Part model, mm, in its own coordinate system. A direction names the side the tool comes from. Give positions to 0.01 mm unless a question says otherwise; leave off trailing zeros. Order: outer loops, then holes, each group sorted by start corner. A loop starts at its lowest first (then second) coordinate and runs counter-clockwise, first axis right, second up. Notation, with made-up numbers: (35, -30.75) - (92, -30.75) arc R10 ccw to (92, -17.75) - close; hole circle Ø3 at (-34, 10). An arc over 180 degrees is marked (long way). One line per item, written item: value.
```python
from build123d import *

# Parameters (mm, degrees)
SKETCH1_R           = 140
BOSS_EXTRUDE1_DEPTH = 300
FILLET1_R           = 4


# Read off the part's stored shape, not the designer's step: Shell1
with BuildPart() as part:
    # Sketch1 → Boss-Extrude1 (new body)
    with BuildSketch(Plane(origin=(0, 0, 0), x_dir=(1, 0, 0), z_dir=(0, 1, 0))):
        with Locations(Location((0, 0, 0), (0, 0, 270))):
            Circle(SKETCH1_R)
    extrude(amount=BOSS_EXTRUDE1_DEPTH)

    # Sketch3 → Cut-Revolve1 (revolve, cut)
    with BuildSketch(Plane.XY, mode=Mode.PRIVATE) as cut_revolve1_sk:
        with BuildLine():
            Line((-107.848101266, -4.321058688), (-131.736864002, 293.320012156))
            ThreePointArc((-131.736864002, 293.320012156), (-133.011114968, 295.939391827), (-135.72404248, 297))
            Line((-135.72404248, 297), (-179.746835443, 297))
            Line((-179.746835443, 297), (-193.472957422, -4.321058688))
            Line((-193.472957422, -4.321058688), (-107.848101266, -4.321058688))
        make_face()
    revolve(cut_revolve1_sk.sketch.rotate(Axis((0, -4.321058688, 0), (0, 1, 0)), 270), axis=Axis((0, -4.321058688, 0), (0, 1, 0)), mode=Mode.SUBTRACT)

    # Fillet1
    fillet1_edges = [part.edges().sort_by_distance(p)[0] for p in [
        (0, 0, 108.194910748),
    ]]
    fillet(fillet1_edges, radius=FILLET1_R)

    # Shell1 outline → Shell1 (revolve, cut)
    with BuildSketch(Plane.XY):
        with BuildLine():
            ThreePointArc((104.503089212, 3), (105.18132109, 3.265152043), (105.499883831, 3.919996961))
            Line((105.499883831, 3.919996961), (128.746480143, 293.560021272))
            ThreePointArc((128.746480143, 293.560021272), (130.976419333, 298.143935697), (135.72404248, 300))
            Line((135.72404248, 300), (0, 300))
            Line((0, 300), (0, 3))
            Line((0, 3), (104.503089212, 3))
        make_face()
    revolve(axis=Axis((0, 0, 0), (0, 1, 0)), mode=Mode.SUBTRACT)


solid = part.part
```
1) Mould opens along X. For faces 4 (the cylindrical face through (-85.19, 298.48, -111.1)), 5 (the flat face through (73, 300, -115)), 6 (the conical face through (-25.425, 150.767, 114.497)) say: released by +X, released by -X, zero draft, split by the parting line, or undercut.
Outcome:
face 4: split by the parting line
face 5: zero draft
face 6: undercut
2) Which spindle directions (+Z, -Z, +X, -X, +Y, -Y) get a long thin tool onto all of the face, cutting with end or side? Do faces 1 (the flat face through (-73, 297, -115)), 2 (the flat face through (1, 0, -1)), 3 (the flat face through (1, 3, -1)). Say none if no direction does.
Outcome:
face 1: -Y
face 2: +Z, -Z, +X, -X, -Y
face 3: +Y
3) Cut at C-C, the plane y = 46. Give the cut face in (x, z), then the cut area to 3 significant figures.
Outcome:
outline: circle Ø223.77 at (0, 0); hole circle Ø217.75 at (0, 0)
area: 2,090 mm^2
4) Cut at B-B, the plane x = 0. Give the cut face in (y, z).
Outcome:
outline: (0, -104.5) arc R4 ccw to (3.68, -108.49) - (293.32, -131.74) arc R4 cw to (297, -135.72) - (297, -140) - (300, -140) - (300, -135.72) arc R7 ccw to (293.56, -128.75) - (3.92, -105.5) arc R1 cw to (3, -104.5) - (3, 104.5) arc R1 cw to (3.92, 105.5) - (293.56, 128.75) arc R7 ccw to (300, 135.72) - (300, 140) - (297, 140) - (297, 135.72) arc R4 cw to (293.32, 131.74) - (3.68, 108.49) arc R4 ccw to (0, 104.5) - close
5) Cut at D-D, the plane y = 171.5. Give the cut face in (x, z), then the cut area to 3 significant figures.
Outcome:
outline: circle Ø243.92 at (0, 0); hole circle Ø237.9 at (0, 0)
area: 2,280 mm^2
6) Drill centre lines: line 1 along Y through (x, z) = (-18.5, -17.5); line 2 along X through (y, z) = (203, -74); line 3 along Z through (x, y) = (-10.5, 93.5). Where is each one in solid material? Low to high. Write a range as from..to.
Outcome:
line 1: y = 0..3
line 2: x = -100.11..-96.34, 96.34..100.11
line 3: z = -115.22..-112.2, 112.2..115.22
7) Pin check, flat tips, straight feed: pin 1 (10 mm diameter, centred on x = 15, z = -8.5, fed in from -Y); pin 2 (3 mm diameter, centred on x = 58, z = -63, fed in from +Y); pin 3 (4 mm diameter, centred on y = 102.5, z = -65, fed in from +X); pin 4 (1 mm diameter, centred on y = 259.5, z = -111, fed in from -X). Stop position of each tip, or through.
Outcome:
pin 1: stops at y = 0
pin 2: stops at y = 3
pin 3: stops at x = 97.92
pin 4: stops at x = -66.61
